```python
from build123d import *

# Parameters (mm, degrees)
HEADFILLET_R     = 0.2
NOTCH_DEPTH      = 20.900217222
NOTCH_DEPTH_BACK = 20.900217222
SKETCH2_W        = 2.3
SKETCH2_H        = 2


with BuildPart() as part:
    # Sketch1 → Base (revolve)
    with BuildSketch(Plane.XY, mode=Mode.PRIVATE) as base_sk:
        Polygon((0, 0), (0, 8.65), (4.65, 4), (16, 4), (16, 0), align=None)
    revolve(base_sk.sketch.rotate(Axis((-5.569640847, 0, 0), (1, 0, 0)), 90), axis=Axis((-5.569640847, 0, 0), (1, 0, 0)))

    # HeadFillet
    headfillet_edges = [part.edges().sort_by_distance(p)[0] for p in [
        (0, 0, -8.65),
    ]]
    fillet(headfillet_edges, radius=HEADFILLET_R)

    # Sketch2 → Notch (cut, two sides: drawn at the far end of the back side and taken through both)
    with BuildSketch(Plane.XY.offset(-NOTCH_DEPTH_BACK)):
        with Locations((1.15, 0)):
            Rectangle(SKETCH2_W, SKETCH2_H)
    extrude(amount=NOTCH_DEPTH + NOTCH_DEPTH_BACK, mode=Mode.SUBTRACT)


solid = part.part
```
Input: part model. Units: mm. Frame: model coordinates. A direction names the side the tool comes from. Give positions to 0.01 mm unless a question says otherwise; leave off trailing zeros. Order: outer loops, then holes, each group sorted by start corner. A loop starts at its lowest first (then second) coordinate and runs counter-clockwise, first axis right, second up. Notation, with made-up numbers: (28.5, 83.5) - (42.5, 83.5) arc R32 ccw to (42.5, 120.5) - close; hole circle Ø10 at (2.25, 69.5). An arc over 180 degrees is marked (long way). Put each result on its own line as item: value.
Item 1: Contact query for flat-ended pins moving along their axis: pin 1 (1 mm diameter, centred on x = 10, z = 1, fed in from -Y); pin 2 (1.2 mm diameter, centred on x = 1, z = 3.5, fed in from +Y); pin 3 (3 mm diameter, centred on x = 14, y = 1, fed in from +Z). Output: stop coordinate, or through.
Found:
pin 1: stops at y = -3.97
pin 2: stops at y = 7.52
pin 3: stops at z = 4
Item 2: Ray query, L1, parallel to X at y = 0.5, z = -0.25; L2, parallel to X at y = -5, z = -3; L3, parallel to Y at x = 10, z = 2.25. Return the intervals inside material, ascending. Write a range as from..to.
Found:
L1: x = 2.3..16
L2: x = 0..2.82
L3: y = -3.31..3.31
Item 3: Draft query along Y for faces 3 (the cylindrical face through (10.404, 3.905, -0.867)), 4 (the flat face through (2.3, 0, 0)), 5 (the flat face through (16, 0, 0)). Return one class per face: +Y half, -Y half, draft (parallel to the pull), parting line (faces both ways), or undercut.
Found:
face 3: parting line
face 4: undercut
face 5: draft
Item 4: Section query C-C, the plane x = 13.75. Return loops of the section in (y, z), then the cut area to 3 significant figures.
Found:
outline: circle Ø8 at (0, 0)
area: 50.3 mm^2
Item 5: Section query B-B, the plane y = 0. Return loops of the section in (x, z), then the cut area to 3 significant figures.
Found:
outline: (2.3, -6.35) - (4.65, -4) - (16, -4) - (16, 4) - (4.65, 4) - (2.3, 6.35) - close
area: 115 mm^2
Item 6: Access query for faces 1 (the conical face through (4.441, -1.264, 4.015)), 2 (the flat face through (1, 1, 0)). Directions: +Z, -Z, +X, -X, +Y, -Y. A direction counts if a zero-diameter tool reaches every point of the face in a straight line with its end or side. Return the directions, or none.
Found:
face 1: +X
face 2: +Z, -Z, -X
Item 7: Section query A-A, the plane z = 0. Return loops of the section in (x, y).
Found:
outline: (0, -8.17) arc R0.2 ccw to (0.34, -8.31) - (4.65, -4) - (16, -4) - (16, 4) - (4.65, 4) - (0.34, 8.31) arc R0.2 ccw to (0, 8.17) - (0, 1) - (2.3, 1) - (2.3, -1) - (0, -1) - close
